Geometry check sheet. Reference: the model listing, model coordinates, mm. A direction names the side the tool comes from. Round coordinates to 2 decimals unless told otherwise and drop trailing zeros. Order: outer loops, then holes, each group sorted by start corner. A loop starts at its lowest first (then second) coordinate and runs counter-clockwise, first axis right, second up. Notation, with made-up numbers: (49, 20.5) - (75, 20.5) arc R16 ccw to (75, 49.5) - close; hole circle Ø7 at (27, 50). An arc over 180 degrees is marked (long way). Return JSON: item names as keys, results as strings. Group by question number.
Q1. Draft check along Y on faces 1 (the flat face through (24.141, 31.725, 1.479)), 2 (the flat face through (58.143, 21, 1)), 3 (the flat face through (29, 0, 3)). Enter one of: pulls with the +Y half, pulls with the -Y half, needs draft (parallel to the pull), parting line crosses it, or undercut.
Q2. Sectioned sample at A-A, the plane z = 2.25. Record the cut outline in (x, y).
Q3. Gauge pin test, flat end, axial feed: pin 1 Ø0.6 at (x, y) = (29.5, 42.5) entering from +Z. Record the tip position at first contact, or that the pin passes through.
Q4. Sectioned sample at B-B, the plane y = 18. Record the cut outline in (x, z).
Q5. Sectioned sample at C-C, the plane x = 54.07. Record the cut outline in (y, z), then the cut area to 3 significant figures.
Q6. Sectioned sample at D-D, the plane y = 28. Record the cut outline in (x, z), then the cut area to 3 significant figures.
Q7. Tool access check on faces 4 (the flat face through (4, 3.8, 5)), 5 (the flat face through (44.51, 29.19, 1.48)), 6 (the flat face through (31.57, 42, 5)), 7 (the cylindrical face through (28.07, 1.34, 5.46)). Record the directions out of +Z, -Z, +X, -X, +Y, -Y that give a thin tool (end or side, any length) a straight path to the whole face; none if there is none.
Q8. Material ranges on line 1 along Y through (x, z) = (29.07, 6.7); line 2 along X through (y, z) = (41.5, 7.25); line 3 along Y through (x, z) = (21.5, 0.75), recorded low to high.
```python
from build123d import *

# Parameters (mm, degrees)
SKETCH1_W           = 58.1426
SKETCH1_H           = 43.5894
BOSS_EXTRUDE1_DEPTH = 3
SKETCH2_R           = 1
BOSS_EXTRUDE2_DEPTH = 5


with BuildPart() as part:
    # Sketch1 → Boss-Extrude1 (new body)
    with BuildSketch(Plane.XY):
        with Locations((29.0713, 21.7947)):
            Rectangle(SKETCH1_W, SKETCH1_H)
        Polygon((6, 36.7947), (6, 6.7947), (21.0529, 21.7947), align=None, mode=Mode.SUBTRACT)
        Polygon((39.0713, 6.7947), (29.0713, 16.7947), (19.0713, 6.7947), align=None, mode=Mode.SUBTRACT)
        Polygon((52.1426, 36.7947), (52.1426, 6.7947), (37.0897, 21.7947), align=None, mode=Mode.SUBTRACT)
        Polygon((19.0713, 36.7947), (39.0713, 36.7947), (29.0713, 26.7947), align=None, mode=Mode.SUBTRACT)
    extrude(amount=BOSS_EXTRUDE1_DEPTH)

    # Sketch2 → Boss-Extrude2 (add)
    with BuildSketch(Plane.XY.offset(3)):
        with BuildLine():
            Line((1.57, 43.5894), (6.57, 43.5894))
            Line((6.57, 43.5894), (6.57, 40.7894))
            ThreePointArc((6.57, 40.7894), (6.277106781, 40.082293219), (5.57, 39.7894))
            Line((5.57, 39.7894), (2.57, 39.7894))
            ThreePointArc((2.57, 39.7894), (1.862893219, 40.082293219), (1.57, 40.7894))
            Line((1.57, 40.7894), (1.57, 43.5894))
        make_face()
        with Locations((4.07, 42.2894)):
            Circle(SKETCH2_R, mode=Mode.SUBTRACT)
        with BuildLine():
            Line((26.57, 43.5894), (31.57, 43.5894))
            Line((31.57, 43.5894), (31.57, 40.7894))
            ThreePointArc((31.57, 40.7894), (31.277106781, 40.082293219), (30.57, 39.7894))
            Line((30.57, 39.7894), (27.57, 39.7894))
            ThreePointArc((27.57, 39.7894), (26.862893219, 40.082293219), (26.57, 40.7894))
            Line((26.57, 40.7894), (26.57, 43.5894))
        make_face()
        with Locations((29.07, 42.2894)):
            Circle(SKETCH2_R, mode=Mode.SUBTRACT)
        with BuildLine():
            Line((51.57, 43.5894), (56.57, 43.5894))
            Line((56.57, 43.5894), (56.57, 40.7894))
            ThreePointArc((56.57, 40.7894), (56.277106781, 40.082293219), (55.57, 39.7894))
            Line((55.57, 39.7894), (52.57, 39.7894))
            ThreePointArc((52.57, 39.7894), (51.862893219, 40.082293219), (51.57, 40.7894))
            Line((51.57, 40.7894), (51.57, 43.5894))
        make_face()
        with Locations((54.07, 42.2894)):
            Circle(SKETCH2_R, mode=Mode.SUBTRACT)
        with BuildLine():
            Line((56.57, 0), (56.57, 2.8))
            ThreePointArc((56.57, 2.8), (56.277106781, 3.507106781), (55.57, 3.8))
            Line((55.57, 3.8), (52.57, 3.8))
            ThreePointArc((52.57, 3.8), (51.862893219, 3.507106781), (51.57, 2.8))
            Line((51.57, 2.8), (51.57, 0))
            Line((51.57, 0), (56.57, 0))
        make_face()
        with Locations((54.07, 1.3)):
            Circle(SKETCH2_R, mode=Mode.SUBTRACT)
        with BuildLine():
            Line((31.57, 0), (31.57, 2.8))
            ThreePointArc((31.57, 2.8), (31.277106781, 3.507106781), (30.57, 3.8))
            Line((30.57, 3.8), (27.57, 3.8))
            ThreePointArc((27.57, 3.8), (26.862893219, 3.507106781), (26.57, 2.8))
            Line((26.57, 2.8), (26.57, 0))
            Line((26.57, 0), (31.57, 0))
        make_face()
        with Locations((29.07, 1.3)):
            Circle(SKETCH2_R, mode=Mode.SUBTRACT)
        with BuildLine():
            Line((6.57, 0), (6.57, 2.8))
            ThreePointArc((6.57, 2.8), (6.277106781, 3.507106781), (5.57, 3.8))
            Line((5.57, 3.8), (2.57, 3.8))
            ThreePointArc((2.57, 3.8), (1.862893219, 3.507106781), (1.57, 2.8))
            Line((1.57, 2.8), (1.57, 0))
            Line((1.57, 0), (6.57, 0))
        make_face()
        with Locations((4.07, 1.3)):
            Circle(SKETCH2_R, mode=Mode.SUBTRACT)
    extrude(amount=BOSS_EXTRUDE2_DEPTH)


solid = part.part
```
Reply:
{
 "1": {"face 1": "undercut", "face 2": "needs draft", "face 3": "pulls with the -Y half"},
 "2": {"outline": "(0, 0) - (58.14, 0) - (58.14, 43.59) - (0, 43.59) - close; hole (6, 6.79) - (21.05, 21.79) - (6, 36.79) - close; hole (19.07, 6.79) - (39.07, 6.79) - (29.07, 16.79) - close; hole (19.07, 36.79) - (29.07, 26.79) - (39.07, 36.79) - close; hole (37.09, 21.79) - (52.14, 6.79) - (52.14, 36.79) - close"},
 "3": {"pin 1": "z = 3"},
 "4": {"outline": "(0, 0) - (6, 0) - (6, 3) - (0, 3) - close; (17.24, 0) - (40.9, 0) - (40.9, 3) - (17.24, 3) - close; (52.14, 0) - (58.14, 0) - (58.14, 3) - (52.14, 3) - close"},
 "5": {"outline": "(0, 0) - (43.59, 0) - (43.59, 8) - (43.29, 8) - (43.29, 3) - (41.29, 3) - (41.29, 8) - (39.79, 8) - (39.79, 3) - (3.8, 3) - (3.8, 8) - (2.3, 8) - (2.3, 3) - (0.3, 3) - (0.3, 8) - (0, 8) - close", "area": "149 mm^2"},
 "6": {"outline": "(0, 0) - (6, 0) - (6, 3) - (0, 3) - close; (14.83, 0) - (27.87, 0) - (27.87, 3) - (14.83, 3) - close; (30.28, 0) - (43.32, 0) - (43.32, 3) - (30.28, 3) - close; (52.14, 0) - (58.14, 0) - (58.14, 3) - (52.14, 3) - close", "area": "114 mm^2"},
 "7": {"face 4": "+Z, +X, -X", "face 5": "+Z, -Z", "face 6": "+Z, +Y, -Y", "face 7": "+Z"},
 "8": {"line 1": "0 to 0.3, 2.3 to 3.8, 39.79 to 41.29, 43.29 to 43.59", "line 2": "1.57 to 3.46, 4.68 to 6.57, 26.57 to 28.46, 29.68 to 31.57, 51.57 to 53.46, 54.68 to 56.57", "line 3": "0 to 6.79, 9.22 to 34.37, 36.79 to 43.59"}
}
